```python
from build123d import *

# Parameters (mm, degrees)
SKETCH_1_W          = 580
SKETCH_1_H          = 560
EXTRUDE_1_DEPTH     = 15
SKETCH_3_W          = 580
SKETCH_3_H          = 500.057079529
EXTRUDE_2_DEPTH     = 15
SKETCH_4_R          = 10
SKETCH_4_W          = 58
SKETCH_4_H          = 70
CUT_EXTRUDE_1_DEPTH = 15
SKETCH_5_W          = 40
SKETCH_5_H          = 40
SKETCH_5_R          = 10
EXTRUDE_3_DEPTH     = 7
SKETCH_6_W          = 100
SKETCH_6_H          = 50
SKETCH_6_R          = 8
EXTRUDE_4_DEPTH     = 10
EXTRUDE_START       = -10
SKETCH_7_W          = 100
SKETCH_7_H          = 50
SKETCH_7_R          = 8
EXTRUDE_5_DEPTH     = 10
SKETCH_8_W          = 580
SKETCH_8_H          = 15
EXTRUDE_6_DEPTH     = 27.2
SKETCH_9_W          = 580
SKETCH_9_H          = 5
EXTRUDE_7_DEPTH     = 550
SKETCH_10_R         = 5
EXTRUDE_8_DEPTH     = 150
SKETCH_11_W         = 360
SKETCH_11_H         = 160
EXTRUDE_9_DEPTH     = 8
SKETCH_12_W         = 30
SKETCH_12_H         = 30
EXTRUDE_10_DEPTH    = 40
SKETCH_13_W         = 30
SKETCH_13_H         = 30
EXTRUDE_11_DEPTH    = 138
SKETCH_14_W         = 127.257079529
SKETCH_14_H         = 70
EXTRUDE_12_DEPTH    = 10
SKETCH_15_R         = 10
SKETCH_15_R_2       = 7
SKETCH_15_R_3       = 2.5
EXTRUDE_13_DEPTH    = 3
FILLET_2_R          = 2
SKETCH_16_R         = 5
EXTRUDE_14_DEPTH    = 20
SKETCH_17_W         = 119.457499099
SKETCH_17_H         = 58.776896967
EXTRUDE_15_DEPTH    = 3
SKETCH_18_W         = 78.016217291
SKETCH_18_H         = 31.996524559
SKETCH_18_R         = 1.406019753
SKETCH_18_R_2       = 1.53736257
SKETCH_18_R_3       = 1.499754403
EXTRUDE_16_DEPTH    = 5


with BuildPart() as part:
    # Sketch 1 → Extrude 1 (new body)
    with BuildSketch(Plane.XY):
        with Locations((200, 280)):
            Rectangle(SKETCH_1_W, SKETCH_1_H)
        Polygon((200, 401.320557861), (350, 401.320557861), (350, 281.320557861), (50, 281.320557861), (50, 401.320557861), align=None, mode=Mode.SUBTRACT)
    extrude(amount=EXTRUDE_1_DEPTH)



with BuildPart() as body_2:
    # Sketch 3 → Extrude 2 (new body)
    with BuildSketch(Plane.XZ):
        with Locations((200, -235.028539765)):
            Rectangle(SKETCH_3_W, SKETCH_3_H)
    extrude(amount=EXTRUDE_2_DEPTH)

    # Sketch 4 → Cut-Extrude 1 (cut)
    with BuildSketch(Plane.XZ.offset(15)):
        with Locations(Location((200, -425.057079529, 0), (0, 0, 270))):
            Circle(SKETCH_4_R)
        with Locations((409, -70.057079529)):
            Rectangle(SKETCH_4_W, SKETCH_4_H)
        with Locations((-9, -70.057079529)):
            Rectangle(SKETCH_4_W, SKETCH_4_H)
    extrude(amount=-CUT_EXTRUDE_1_DEPTH, mode=Mode.SUBTRACT)

    # Sketch 5 → Extrude 3 (add)
    with BuildSketch(Plane.XZ.offset(15)):
        with Locations((200, -425.057079529)):
            Rectangle(SKETCH_5_W, SKETCH_5_H)
        with Locations(Location((200, -425.057079529, 0), (0, 0, 270))):
            Circle(SKETCH_5_R, mode=Mode.SUBTRACT)
    extrude(amount=EXTRUDE_3_DEPTH)


with BuildPart() as part_1:
    add(part.part)

    add(body_2.part)  # Extrude 4 merges body 2
    # Sketch 6 → Extrude 4 (add)
    with BuildSketch(Plane.ZY.offset(90)):
        with Locations((-50, 25)):
            Rectangle(SKETCH_6_W, SKETCH_6_H)
        with Locations((-50, 25)):
            Circle(SKETCH_6_R, mode=Mode.SUBTRACT)
    extrude(amount=-EXTRUDE_4_DEPTH)

    # Sketch 7 → Extrude 5 (add)
    with BuildSketch(Plane(origin=(490, 0, 0), x_dir=(0, 0, -1), z_dir=(1, 0, 0)).offset(EXTRUDE_START)):
        with Locations((50, 25)):
            Rectangle(SKETCH_7_W, SKETCH_7_H)
        with Locations(Location((50, 25, 0), (0, 0, 180))):
            Circle(SKETCH_7_R, mode=Mode.SUBTRACT)
    extrude(amount=EXTRUDE_5_DEPTH)

    # Sketch 8 → Extrude 6 (add)
    with BuildSketch(Plane(origin=(0, 0, -485.057079529), x_dir=(-1, 0, 0), z_dir=(0, 0, -1))):
        with Locations((-200, -7.5)):
            Rectangle(SKETCH_8_W, SKETCH_8_H)
    extrude(amount=EXTRUDE_6_DEPTH)

    # Sketch 9 → Extrude 7 (add)
    with BuildSketch(Plane(origin=(0, 0, 0), x_dir=(1, 0, 0), z_dir=(0, 1, 0))):
        with Locations((200, 509.757079529)):
            Rectangle(SKETCH_9_W, SKETCH_9_H)
    extrude(amount=EXTRUDE_7_DEPTH)

    # Sketch 10 → Extrude 8 (add)
    with BuildSketch(Plane(origin=(0, 0, 0), x_dir=(1, 0, 0), z_dir=(0, 1, 0))):
        with Locations(Location((10, 387.257079529, 0), (0, 0, 270))):
            Circle(SKETCH_10_R)
        with Locations(Location((330, 387.257079529, 0), (0, 0, 270))):
            Circle(SKETCH_10_R)
        with Locations(Location((10, 267.257079529, 0), (0, 0, 270))):
            Circle(SKETCH_10_R)
        with Locations(Location((330, 267.257079529, 0), (0, 0, 270))):
            Circle(SKETCH_10_R)
    extrude(amount=EXTRUDE_8_DEPTH)

    # Sketch 11 → Extrude 9 (add)
    with BuildSketch(Plane(origin=(0, 150, 0), x_dir=(1, 0, 0), z_dir=(0, 1, 0))):
        with Locations((170, 327.257079529)):
            Rectangle(SKETCH_11_W, SKETCH_11_H)
    extrude(amount=EXTRUDE_9_DEPTH)

    # Sketch 12 → Extrude 10 (add)
    with BuildSketch(Plane(origin=(0, 158, 0), x_dir=(1, 0, 0), z_dir=(0, 1, 0))):
        with Locations((113, 349.257079529)):
            Rectangle(SKETCH_12_W, SKETCH_12_H)
    extrude(amount=EXTRUDE_10_DEPTH)

    # Sketch 13 → Extrude 11 (add)
    with BuildSketch(Plane(origin=(0, 158, 0), x_dir=(1, 0, 0), z_dir=(0, 1, 0))):
        with Locations((326, 358.257079529)):
            Rectangle(SKETCH_13_W, SKETCH_13_H)
    extrude(amount=EXTRUDE_11_DEPTH)

    # Sketch 14 → Extrude 12 (add)
    with BuildSketch(Plane.ZY.offset(90)):
        with Locations((-263.628539765, 35)):
            Rectangle(SKETCH_14_W, SKETCH_14_H)
    extrude(amount=-EXTRUDE_12_DEPTH)

    # Sketch 15 → Extrude 13 (add)
    # profile 1 of 2: a face of its own
    with BuildSketch(Plane.ZY.offset(90)):
        with Locations(Location((-263.628539764, 35, 0), (0, 0, 180))):
            Circle(SKETCH_15_R)
        with Locations((-263.628539764, 35)):
            Circle(SKETCH_15_R_2, mode=Mode.SUBTRACT)
    # profile 2 of 2: a face of its own
    with BuildSketch(Plane.ZY.offset(90)):
        with Locations(Location((-263.628539764, 35, 0), (0, 0, 180))):
            Circle(SKETCH_15_R_3)
    extrude(amount=EXTRUDE_13_DEPTH)

    # Fillet 2
    fillet_2_edges = [part_1.edges().sort_by_distance(p)[0] for p in [
        (-93, 35, -253.628539764),
        (-93, 35, -261.128539764),
    ]]
    fillet(fillet_2_edges, radius=FILLET_2_R)

    # Sketch 16 → Extrude 14 (add)
    with BuildSketch(Plane(origin=(0, 158, 0), x_dir=(1, 0, 0), z_dir=(0, 1, 0))):
        with Locations(Location((171.790204926, 271.64043121, 0), (0, 0, 270))):
            Circle(SKETCH_16_R)
        with Locations(Location((270.129191609, 271.64043121, 0), (0, 0, 270))):
            Circle(SKETCH_16_R)
        with Locations(Location((171.790204926, 310.918685367, 0), (0, 0, 270))):
            Circle(SKETCH_16_R)
        with Locations(Location((270.129191609, 310.918685367, 0), (0, 0, 270))):
            Circle(SKETCH_16_R)
    extrude(amount=EXTRUDE_14_DEPTH)

    # Sketch 17 → Extrude 15 (add)
    with BuildSketch(Plane(origin=(0, 178, 0), x_dir=(1, 0, 0), z_dir=(0, 1, 0))):
        with Locations((220.921909881, 290.395031068)):
            Rectangle(SKETCH_17_W, SKETCH_17_H)
    extrude(amount=EXTRUDE_15_DEPTH)

    # Sketch 18 → Extrude 16 (add)
    with BuildSketch(Plane(origin=(0, 181, 0), x_dir=(1, 0, 0), z_dir=(0, 1, 0))):
        with Locations((219.405209005, 291.746230642)):
            Rectangle(SKETCH_18_W, SKETCH_18_H)
        with Locations(Location((184.299854938, 304.10663833, 0), (0, 0, 270))):
            Circle(SKETCH_18_R, mode=Mode.SUBTRACT)
        with Locations(Location((184.299854938, 278.517078822, 0), (0, 0, 270))):
            Circle(SKETCH_18_R_2, mode=Mode.SUBTRACT)
        with Locations(Location((254.507107947, 278.517078822, 0), (0, 0, 270))):
            Circle(SKETCH_18_R_3, mode=Mode.SUBTRACT)
    extrude(amount=EXTRUDE_16_DEPTH)


solid = part_1.part
```
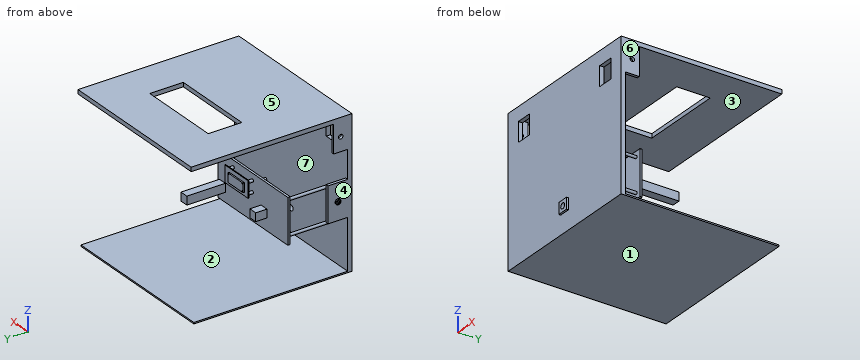
The listing builds one solid part. Answer for the finished solid, in the listing's coordinates (mm). Face numbers are marked on the shaded views. A direction names the side the tool comes from. Give positions to 0.01 mm unless a question says otherwise; leave off trailing zeros. Order: outer loops, then holes, each group sorted by start corner. A loop starts at its lowest first (then second) coordinate and runs counter-clockwise, first axis right, second up. Notation, with made-up numbers: (-33.5, -35.5) -> (-9.5, -35.5) arc R16 ccw to (-9.5, -14.5) -> close; hole circle Ø4 at (8, 4). An arc over 180 degrees is marked (long way). Write each question's results on one line, items separated by ' | '.
Q1. The part is cut by section C-C, the plane x = 200. State how many separate pieces and enclosed holes the cut face has, and give its area (3 significant figures).
Checked values:
separate pieces: 5 | enclosed holes: 0 | area: 18,700 mm^2
Q2. Determine the mould class of the marked faces 4, 5, 6 and 7 for opening direction X: pulls with the +X half, pulls with the -X half, needs draft (parallel to the pull), parting line crosses it, or undercut.
Checked values:
face 4: pulls with the -X half | face 5: needs draft | face 6: pulls with the +X half | face 7: undercut
Q3. The part is cut by section A-A, the plane y = 83.5. Give the vertices of the cut face in (x, z).
Checked values:
outline: (-90, -512.26) -> (490, -512.26) -> (490, -507.26) -> (-90, -507.26) -> close; (-90, 0) -> (490, 0) -> (490, 15) -> (-90, 15) -> close; circle Ø10 at (10, -387.26); circle Ø10 at (10, -267.26); circle Ø10 at (330, -387.26); circle Ø10 at (330, -267.26)
Q4. Straight lines are drawn through the part: probe 1 along Z at (x, y) = (485, 25); probe 2 along Z at (x, y) = (344.5, 490.5); probe 3 along Y at (x, z) = (226.5, -298.5). For each, find the intervals that lie inside material, in ascending order. Write a range as from..to.
Checked values:
probe 1: z = -512.26..-507.26, -100..-58, -42..15 | probe 2: z = -512.26..-507.26, 0..15 | probe 3: y = -15..0, 150..158, 178..186
Q5. Each of these flat-tipped pins is pushed along its axis until it touches: P1, Ø6, axis at x = 281, z = -298.5, coming from the -Y side; P2, Ø4, axis at x = 230, z = -511, coming from the +Y side; P3, Ø7.5, axis at y = -17, z = -421.5, coming from the -X side. Where does it stop, or does it pass through?
Checked values:
P1: stops at y = -15 | P2: stops at y = 550 | P3: stops at x = -90
Q6. The part is cut by section D-D, the plane y = 242. Give the vertices of the cut face in (x, z), and give its area (3 significant figures).
Checked values:
outline: (-90, -512.26) -> (490, -512.26) -> (490, -507.26) -> (-90, -507.26) -> close; (-90, 0) -> (490, 0) -> (490, 15) -> (-90, 15) -> close; (311, -373.26) -> (341, -373.26) -> (341, -343.26) -> (311, -343.26) -> close | area: 12,500 mm^2
Q7. The part is cut by section B-B, the plane z = -50. Give the vertices of the cut face in (x, y).
Checked values:
outline: (-90, -15) -> (-38, -15) -> (-38, 0) -> (-80, 0) -> (-80, 17) -> (-90, 17) -> close; (-90, 33) -> (-80, 33) -> (-80, 50) -> (-90, 50) -> close; (20, -15) -> (380, -15) -> (380, 0) -> (20, 0) -> close; (438, -15) -> (490, -15) -> (490, 17) -> (480, 17) -> (480, 0) -> (438, 0) -> close; (480, 33) -> (490, 33) -> (490, 50) -> (480, 50) -> close
Q8. Which of the six approach directions +Z, -Z, +X, -X, +Y, -Y give full straight-line access (tool end or side, diameter ignored) to the marked faces 1, 2 and 3?
Checked values:
face 1: -Z, +X, -X, +Y, -Y | face 2: +X, -X, +Y | face 3: +Y
